Autodesk Inventor part; units mm, degrees
ref_plane "YZ Plane" through (0, 0, 0) normal (1, 0, 0) x (0, 1, 0)
ref_plane "XZ Plane" through (0, 0, 0) normal (0, 1, 0) x (-1, 0, 0)
ref_plane "XY Plane" through (0, 0, 0) normal (0, 0, 1) x (1, 0, 0)
sketch "Sketch1" plane through (0, 0, 0) normal (0, 0, 1) x (1, 0, 0)
  circle A0 centre (0, 0) radius 7.5
  dimension "d0" = 15
extrude "Extrusion1" add sketch "Sketch1" along normal blind 38
sketch "Sketch2" plane through (0, 0, 38) normal (0, 0, 1) x (1, 0, 0)
  circle A0 centre (0, 0) radius 10
  dimension "d3" = 20
extrude "Extrusion2" add sketch "Sketch2" along normal blind 5
sketch "Sketch5" plane through (0, 0, 43) normal (0, 0, 1) x (1, 0, 0)
  circle A0 centre (0, 0) radius 10
  circle A1 centre (0, 0) radius 5
  dimension "d12" = 10
extrude "Extrusion5" cut sketch "Sketch5" against normal through all contours A1
properties part number "Top"
For this review, take the finished solid that the model builds, in its own axes (mm). A direction names the side the tool comes from. Round coordinates to 2 decimals unless told otherwise and drop trailing zeros. Order: outer loops, then holes, each group sorted by start corner. A loop starts at its lowest first (then second) coordinate and runs counter-clockwise, first axis right, second up. Notation, with made-up numbers: M -33,84 L -26,84 A17 ccw -26,112 Z; hole C 61.5,78 d6. An arc over 180 degrees is marked long. Use a Markdown table: item, result. Add a question column.
Item 1: Add section D-D, the plane x = 6. Give the boundary of the cut face in (y, z), then the cut area to 3 significant figures.
Item 2: To check wall thickness, follow line 1 along Y through (x, z) = (0, 17.5); line 2 along X through (y, z) = (0.75, 26); line 3 along X through (y, z) = (0.5, 41). State the ranges of each line that lie inside material, in increasing order.
Item 3: Add section C-C, the plane z = 37. Give the boundary of the cut face in (x, y).
Item 4: Insertion check: pin 1 (1 mm diameter, centred on x = 2.5, z = 4.5, fed in from +Y); pin 2 (4 mm diameter, centred on y = -1.5, z = 27, fed in from +X); pin 3 (10 mm diameter, centred on y = -1, z = 16, fed in from -X). Each pin has a flat end and moves straight along its axis. Give the tip position at first contact, or say it passes through.
Item 5: Mouldability with a two-part tool opening along Y and no side actions: class faces 3 (the cylindrical face through (-2.17, 9.76, 40.47)), 4 (the flat face through (2, -5, 0)), 5 (the cylindrical face through (-1.08, -4.88, 21.8)) as released by +Y, released by -Y, zero draft, split by the parting line, or undercut.
Item 6: Tool access review of faces 1 (the cylindrical face through (-7.493, -0.33, 18.734)), 2 (the flat face through (2, 5, 43)): name each direction out of +Z, -Z, +X, -X, +Y, -Y from which nothing blocks a thin tool from reaching the whole face with its end or side.
Item 7: Add section B-B, the plane y = -4.5. Give the boundary of the cut face in (x, z).
Item 8: Add section A-A, the plane x = 0. Give the boundary of the cut face in (y, z), then the cut area to 3 significant figures.
Geometry results:
| question | item | result |
|---|---|---|
| 1 | outline | M -8,38 L -4.5,38 L -4.5,0 L 4.5,0 L 4.5,38 L 8,38 L 8,43 L -8,43 Z |
| 1 | area | 422 mm² |
| 2 | line 1 | y = -7.5 to -5, 5 to 7.5 |
| 2 | line 2 | x = -7.46 to -4.94, 4.94 to 7.46 |
| 2 | line 3 | x = -9.99 to -4.97, 4.97 to 9.99 |
| 3 | outline | C 0,0 d15; hole C 0,0 d10 |
| 4 | pin 1 | stops at y = 7.23 |
| 4 | pin 2 | stops at x = 7.5 |
| 4 | pin 3 | stops at x = -7.5 |
| 5 | face 3 | split by the parting line |
| 5 | face 4 | zero draft |
| 5 | face 5 | undercut |
| 6 | face 1 | -Z |
| 6 | face 2 | +Z, +X, -X, +Y, -Y |
| 7 | outline | M -8.93,38 L -6,38 L -6,0 L -2.18,0 L -2.18,43 L -8.93,43 Z; M 2.18,0 L 6,0 L 6,38 L 8.93,38 L 8.93,43 L 2.18,43 Z |
| 8 | outline | M -10,38 L -7.5,38 L -7.5,0 L -5,0 L -5,43 L -10,43 Z; M 5,0 L 7.5,0 L 7.5,38 L 10,38 L 10,43 L 5,43 Z |
| 8 | area | 240 mm² |
